Work out the finished part from the listing and answer in its coordinate system (mm). Give positions to 0.01 mm unless a question says otherwise; leave off trailing zeros. Loops run counter-clockwise (first coordinate to the right, second up) from the corner with the lowest first, then second, coordinate; pieces in that order, holes last. Notation, with made-up numbers: M 33,32.25 L 77,32.25 A3 cw 77,37.25 Z; hole C -28,73 d5. An arc over 180 degrees is marked long. Use a Markdown table: item, result.
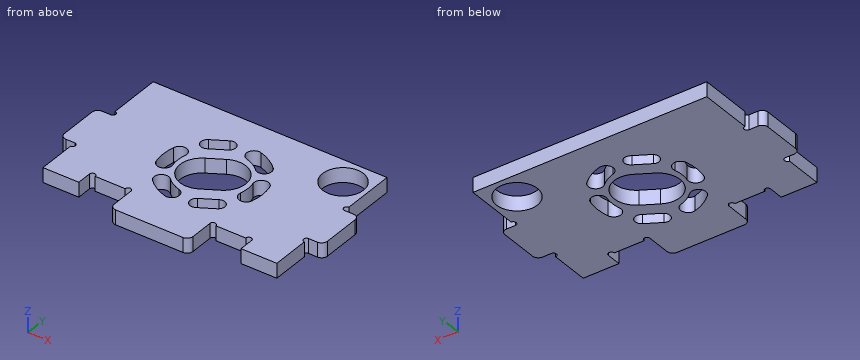
```python
from build123d import *

# Parameters (mm, degrees)
SKETCH_1_W          = 80
SKETCH_1_H          = 52
EXTRUDE_1_DEPTH     = 5
CUT_EXTRUDE_1_DEPTH = 5
SKETCH_3_R          = 7
CUT_EXTRUDE_2_DEPTH = 10
SKETCH_10_W         = 27
SKETCH_10_H         = 5
SKETCH_10_W_2       = 5
SKETCH_10_H_2       = 17
EXTRUDE_3_DEPTH     = 5
SKETCH_11_R         = 1
CUT_EXTRUDE_5_DEPTH = 5
FILLET_1_R          = 2
SKETCH_12_W         = 14.25
SKETCH_12_H         = 5
CUT_EXTRUDE_6_DEPTH = 10
SKETCH_15_R         = 1
CUT_EXTRUDE_7_DEPTH = 10


with BuildPart() as part:
    # 스케치1 → 보스-돌출1 (new body)
    with BuildSketch(Plane.XY):
        with Locations((-2.598076211, 25)):
            Rectangle(SKETCH_1_W, SKETCH_1_H)
        with BuildLine():
            Line((-8.996152423, 29.081793069), (-3.8, 32.081793069))
            ThreePointArc((-3.8, 32.081793069), (6.581793069, 29.3), (3.8, 18.918206931))
            Line((3.8, 18.918206931), (-1.396152423, 15.918206931))
            ThreePointArc((-1.396152423, 15.918206931), (-11.777945491, 18.7), (-8.996152423, 29.081793069))
        make_face(mode=Mode.SUBTRACT)
        with BuildLine():
            ThreePointArc((9.118681917, 36.317368995), (5.799069268, 38.781337822), (1.982863658, 40.371163365))
            ThreePointArc((1.982863658, 40.371163365), (-1.098327994, 38.637306968), (0.635528403, 35.556115316))
            ThreePointArc((0.635528403, 35.556115316), (3.329320598, 34.433885521), (5.672576585, 32.694613408))
            ThreePointArc((5.672576585, 32.694613408), (9.207007044, 32.782938536), (9.118681917, 36.317368995))
        make_face(mode=Mode.SUBTRACT)
        with BuildLine():
            ThreePointArc((13.92745731, 27.988325692), (14.401510584, 23.881472394), (13.870237087, 19.781628618))
            ThreePointArc((13.870237087, 19.781628618), (10.828077575, 17.980166572), (9.026615528, 21.022326083))
            ThreePointArc((9.026615528, 21.022326083), (9.401632115, 23.916333454), (9.067006275, 26.815288723))
            ThreePointArc((9.067006275, 26.815288723), (10.910713308, 29.832032725), (13.92745731, 27.988325692))
        make_face(mode=Mode.SUBTRACT)
        with BuildLine():
            ThreePointArc((-14.31483434, 11.682631005), (-10.995221691, 9.218662178), (-7.179016081, 7.628836635))
            ThreePointArc((-7.179016081, 7.628836635), (-4.097824429, 9.362693032), (-5.831680825, 12.443884684))
            ThreePointArc((-5.831680825, 12.443884684), (-8.52547302, 13.566114479), (-10.868729008, 15.305386592))
            ThreePointArc((-10.868729008, 15.305386592), (-14.403159467, 15.217061464), (-14.31483434, 11.682631005))
        make_face(mode=Mode.SUBTRACT)
        with BuildLine():
            ThreePointArc((-19.123609733, 20.011674308), (-19.597663007, 24.118527606), (-19.066389509, 28.218371382))
            ThreePointArc((-19.066389509, 28.218371382), (-16.024229998, 30.019833428), (-14.222767951, 26.977673917))
            ThreePointArc((-14.222767951, 26.977673917), (-14.597784537, 24.083666546), (-14.263158697, 21.184711277))
            ThreePointArc((-14.263158697, 21.184711277), (-16.106865731, 18.167967275), (-19.123609733, 20.011674308))
        make_face(mode=Mode.SUBTRACT)
    extrude(amount=EXTRUDE_1_DEPTH)

    # 스케치2 → 컷-돌출1 (cut)
    with BuildSketch(Plane.XY.offset(5)):
        with BuildLine():
            Line((8.375, 10.994074487), (3.178847577, 7.994074487))
            ThreePointArc((3.178847577, 7.994074487), (0.105290419, 8.817631645), (0.928847577, 11.891188804))
            Line((0.928847577, 11.891188804), (6.125, 14.891188804))
            ThreePointArc((6.125, 14.891188804), (9.198557159, 14.067631645), (8.375, 10.994074487))
        make_face()
        with BuildLine():
            Line((-6.125, 36.108811196), (-11.321152423, 33.108811196))
            ThreePointArc((-11.321152423, 33.108811196), (-14.394709581, 33.932368355), (-13.571152423, 37.005925513))
            Line((-13.571152423, 37.005925513), (-8.375, 40.005925513))
            ThreePointArc((-8.375, 40.005925513), (-5.301442841, 39.182368355), (-6.125, 36.108811196))
        make_face()
    extrude(amount=-CUT_EXTRUDE_1_DEPTH, mode=Mode.SUBTRACT)

    # 스케치3 → 컷-돌출2 (cut)
    with BuildSketch(Plane.XY.offset(5)):
        with Locations((28.795344676, 42.125)):
            Circle(SKETCH_3_R)
    extrude(amount=-CUT_EXTRUDE_2_DEPTH, mode=Mode.SUBTRACT)

    # 스케치10 → 보스-돌출3 (add)
    with BuildSketch(Plane.XY.offset(5)):
        with Locations((-2.598076211, -3.5)):
            Rectangle(SKETCH_10_W, SKETCH_10_H)
        with Locations((39.901923789, 22.5)):
            Rectangle(SKETCH_10_W_2, SKETCH_10_H_2)
        with Locations((-45.098076211, 22.5)):
            Rectangle(SKETCH_10_W_2, SKETCH_10_H_2)
    extrude(amount=-EXTRUDE_3_DEPTH)

    # 스케치11 → 컷-돌출5 (cut)
    with BuildSketch(Plane.XY.offset(5)):
        with Locations((37.401923789, 32)):
            Circle(SKETCH_11_R)
        with Locations((37.401923789, 13)):
            Circle(SKETCH_11_R)
        with Locations((-42.598076211, 13)):
            Circle(SKETCH_11_R)
        with Locations((-42.598076211, 32)):
            Circle(SKETCH_11_R)
        with Locations((11.901923789, -1)):
            Circle(SKETCH_11_R)
        with Locations((-17.098076211, -1)):
            Circle(SKETCH_11_R)
    extrude(amount=-CUT_EXTRUDE_5_DEPTH, mode=Mode.SUBTRACT)

    # 필렛1
    fillet_1_edges = [part.edges().sort_by_distance(p)[0] for p in [
        (42.401923789, 31, 2.5),
        (42.401923789, 14, 2.5),
        (10.901923789, -6, 2.5),
        (-16.098076211, -6, 2.5),
        (-47.598076211, 14, 2.5),
        (-47.598076211, 31, 2.5),
    ]]
    fillet(fillet_1_edges, radius=FILLET_1_R)

    # 스케치12 → 컷-돌출6 (cut)
    with BuildSketch(Plane.XY.offset(5)):
        with Locations((18.026923789, 1.5)):
            Rectangle(SKETCH_12_W, SKETCH_12_H)
        with Locations((-23.223076211, 1.5)):
            Rectangle(SKETCH_12_W, SKETCH_12_H)
    extrude(amount=-CUT_EXTRUDE_6_DEPTH, mode=Mode.SUBTRACT)

    # 스케치15 → 컷-돌출7 (cut)
    with BuildSketch(Plane.XY.offset(5)):
        with Locations((11.901923789, 4)):
            Circle(SKETCH_15_R)
        with Locations((24.151923789, 4)):
            Circle(SKETCH_15_R)
        with Locations((-17.098076211, 4)):
            Circle(SKETCH_15_R)
        with Locations((-29.348076211, 4)):
            Circle(SKETCH_15_R)
    extrude(amount=-CUT_EXTRUDE_7_DEPTH, mode=Mode.SUBTRACT)


solid = part.part
```
(1) A cutting plane is placed at B-B (x = 17.5). Write down the section's boundary in (y, z).
Entries:
| item | result |
|---|---|
| outline | M 4,0 L 51,0 L 51,5 L 4,5 Z |
(2) Consider probe 1 along X at (y, z) = (0, 0.3); probe 2 along Y at (x, z) = (5.5, 0.9) (3 decimals); probe 3 along Y at (x, z) = (-11, 1.7). Determine where each line is inside the solid, lowest interval first. Write a range as [from, to].
Entries:
| item | result |
|---|---|
| probe 1 | x = [-42.6, -30.35], [-16.1, 10.9], [25.15, 37.4] |
| probe 2 | y = [-6, 9.334], [14.53, 20.255], [30.745, 32.856], [38.947, 51] |
| probe 3 | y = [-6, 9.22], [15.42, 17.59], [27.41, 33.29], [38.49, 51] |
(3) A cutting plane is placed at C-C (z = 2.65). Count the separate pieces of the cut face and the enclosed holes in it, and give its area (3 significant figures).
Entries:
| item | result |
|---|---|
| separate pieces | 1 |
| enclosed holes | 8 |
| area | 3,570 mm² |
(4) Given P1, Ø1.5, axis at x = 39, z = 2, coming from the +Y side; P2, Ø2.5, axis at y = 1.5, z = 2.5, coming from the -X side; P3, Ø1.5, axis at x = 18, z = 3.5, coming from the -Y side, each flat-ended and moving along its own axis, determine where each tip first touches the part or whether it passes through.
Entries:
| item | result |
|---|---|
| P1 | stops at y = 31 |
| P2 | stops at x = -42.6 |
| P3 | stops at y = 4 |
(5) A cutting plane is placed at D-D (y = 39). Write down the section's boundary in (x, z), and give its area (3 significant figures).
Entries:
| item | result |
|---|---|
| outline | M -42.6,0 L -10.12,0 L -10.12,5 L -42.6,5 Z; M -5.21,0 L -0.97,0 L -0.97,5 L -5.21,5 Z; M 5.4,0 L 22.53,0 L 22.53,5 L 5.4,5 Z; M 35.06,0 L 37.4,0 L 37.4,5 L 35.06,5 Z |
| area | 281 mm² |
(6) A cutting plane is placed at A-A (y = 22.5). Write down the section's boundary in (x, z), and give its area (3 significant figures).
Entries:
| item | result |
|---|---|
| outline | M -47.6,0 L -19.53,0 L -19.53,5 L -47.6,5 Z; M -14.5,0 L -12.8,0 L -12.8,5 L -14.5,5 Z; M 6.98,0 L 9.31,0 L 9.31,5 L 6.98,5 Z; M 14.34,0 L 42.4,0 L 42.4,5 L 14.34,5 Z |
| area | 301 mm² |
